The listing builds one solid part. Answer for the finished solid, in the listing's coordinates (mm). Face numbers are marked on the shaded views. A direction names the side the tool comes from. Round coordinates to 2 decimals unless told otherwise and drop trailing zeros. Loops run counter-clockwise (first coordinate to the right, second up) from the corner with the lowest first, then second, coordinate; pieces in that order, holes last. Notation, with made-up numbers: M 29,-13 L 59,-13 A19 ccw 59,3 Z; hole C -23.5,-9.5 d4. An arc over 180 degrees is marked long. Answer as a JSON object with one key per item and string values.
```python
from build123d import *

# Parameters (mm, degrees)
BOX002_W          = 3.6
BOX002_H          = 65
BOX002_DEPTH      = 10
CYLINDER004_R     = 1.8
CYLINDER004_DEPTH = 10
ARRAY_Y_COUNT     = 2
ARRAY_Y_PITCH     = 65
BOX004_W          = 15
BOX004_H          = 29
BOX004_DEPTH      = 10
BOX003_W          = 9.6
BOX003_H          = 65
BOX003_DEPTH      = 4
BOX005_W          = 20
BOX005_H          = 46
BOX005_DEPTH      = 4
CYLINDER006_W     = 23
CYLINDER006_H     = 4
CYLINDER006_ANGLE = 180
CYLINDER005_R     = 4.8
CYLINDER005_DEPTH = 4
ARRAY001_Y_COUNT  = 2
ARRAY001_Y_PITCH  = 65


with BuildPart() as cube002:
    # Box002 → Box002 (new body)
    with BuildSketch(Plane(origin=(-1.8, -32.5, 0), x_dir=(1, 0, 0), z_dir=(0, 0, 1))):
        with Locations((1.8, 32.5)):
            Rectangle(BOX002_W, BOX002_H)
    extrude(amount=BOX002_DEPTH)


with BuildPart() as bolt_hole_fusion:
    # Cylinder004 → Cylinder004 (new body)
    with BuildSketch(Plane.XY):
        Circle(CYLINDER004_R)
    extrude(amount=CYLINDER004_DEPTH)

    # Array Y: bolt hole fusion ×2


with BuildPart() as bolt_hole_fusion_1:
    add(bolt_hole_fusion.part)
    with Locations(*[(0, i * ARRAY_Y_PITCH, 0) for i in range(1, ARRAY_Y_COUNT)]):
        add(bolt_hole_fusion.part)


with BuildPart() as bolt_hole_fusion_2:
    # Array placement: moved
    add(bolt_hole_fusion_1.part.moved(Location((0, -32.5, 0))))

    # Fusion003: union Cube002
    add(cube002.part)


with BuildPart() as extract_fusion:
    # Box004 → Box004 (new body)
    with BuildSketch(Plane(origin=(-8, -14, 0), x_dir=(1, 0, 0), z_dir=(0, 0, 1))):
        with Locations((7.5, 14.5)):
            Rectangle(BOX004_W, BOX004_H)
    extrude(amount=BOX004_DEPTH)

    # Fusion005: union bolt hole fusion
    add(bolt_hole_fusion_2.part)


with BuildPart() as wall_cube:
    # Box003 → Box003 (new body)
    with BuildSketch(Plane(origin=(-4.8, -32.5, 0), x_dir=(1, 0, 0), z_dir=(0, 0, 1))):
        with Locations((4.8, 32.5)):
            Rectangle(BOX003_W, BOX003_H)
    extrude(amount=BOX003_DEPTH)


with BuildPart() as obj1:
    # Box005 → Box005 (new body)
    with BuildSketch(Plane(origin=(-10, -23, 0), x_dir=(1, 0, 0), z_dir=(0, 0, 1))):
        with Locations((10, 23)):
            Rectangle(BOX005_W, BOX005_H)
    extrude(amount=BOX005_DEPTH)


with BuildPart() as cover_cylinder:
    # Cylinder006 → Cylinder006 (revolve)
    with BuildSketch(Plane(origin=(10, 0, 0), x_dir=(0, -1, 0), z_dir=(-1, 0, 0))):
        with Locations((11.5, 2)):
            Rectangle(CYLINDER006_W, CYLINDER006_H)
    revolve(axis=Axis((10, 0, 0), (0, 0, 1)), revolution_arc=CYLINDER006_ANGLE)


with BuildPart() as part_mirroring:
    # Part__Mirroring: instance of cover cylinder
    add(cover_cylinder.part.mirror(Plane(origin=(0, 0, 0), x_dir=(0, -1, 0), z_dir=(1, 0, 0))))


with BuildPart() as microscope_attachment_cut:
    # Cylinder005 → Cylinder005 (new body)
    with BuildSketch(Plane.XY):
        Circle(CYLINDER005_R)
    extrude(amount=CYLINDER005_DEPTH)

    # Array001 Y: microscope attachment cut ×2


with BuildPart() as microscope_attachment_cut_1:
    add(microscope_attachment_cut.part)
    with Locations(*[(0, i * ARRAY001_Y_PITCH, 0) for i in range(1, ARRAY001_Y_COUNT)]):
        add(microscope_attachment_cut.part)


with BuildPart() as microscope_attachment_cut_2:
    # Array001 placement: moved
    add(microscope_attachment_cut_1.part.moved(Location((0, -32.5, 0))))

    # Fusion004: union wall cube, obj1, Part__Mirroring, cover cylinder
    add(wall_cube.part)
    add(obj1.part)
    add(part_mirroring.part)
    add(cover_cylinder.part)

    # Cut001: cut extract fusion
    add(extract_fusion.part, mode=Mode.SUBTRACT)


solid = microscope_attachment_cut_2.part
```
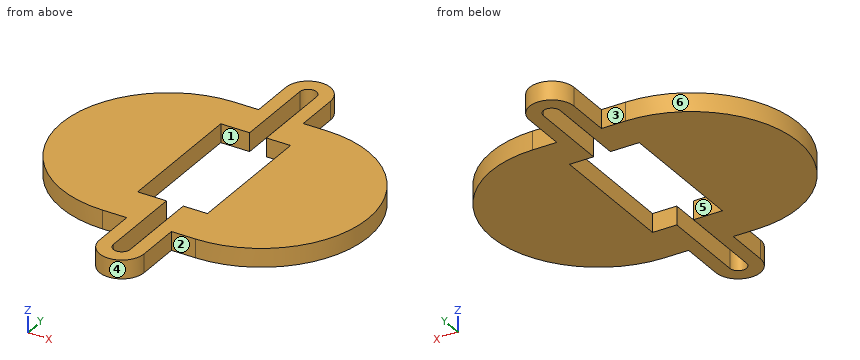
Item 1: Which of the six approach directions +Z, -Z, +X, -X, +Y, -Y give full straight-line access (tool end or side, diameter ignored) to the marked faces 1, 2 and 3?
Values follow:
{"face 1": "+Z, -Z", "face 2": "+Z, -Z, +X, -Y", "face 3": "+Z, -Z, -X, +Y"}
Item 2: The part is cut by section C-C (z = 1.9). Give the vertices of the cut face in (x, y).
Values follow:
{"outline": "M -10,-23 L -4.8,-23 L -4.8,-32.5 A4.8 ccw 4.8,-32.5 L 4.8,-23 L 10,-23 A23 ccw 10,23 L 4.8,23 L 4.8,32.5 A4.8 ccw -4.8,32.5 L -4.8,23 L -10,23 A23 ccw Z; hole M -8,-14 L -1.8,-14 L -1.8,-32.5 A1.8 ccw 1.8,-32.5 L 1.8,-14 L 7,-14 L 7,15 L 1.8,15 L 1.8,32.5 A1.8 ccw -1.8,32.5 L -1.8,15 L -8,15 Z"}
Item 3: The part is cut by section D-D (x = 24.5). Give the vertices of the cut face in (y, z).
Values follow:
{"outline": "M -17.85,0 L 17.85,0 L 17.85,4 L -17.85,4 Z"}
Item 4: Straight lines are drawn through the part: line 1 (X direction, y = 32, z = 1.5); line 2 (Y direction, x = 5, z = 1); line 3 (X direction, y = -15, z = 2.2). For each, find the intervals that lie inside material, in ascending order.
Values follow:
{"line 1": "-4.8 to -1.8, 1.8 to 4.8", "line 2": "-23 to -14, 15 to 23", "line 3": "-27.44 to -1.8, 1.8 to 27.44"}
Item 5: The part is cut by section A-A (y = -31.5). Give the vertices of the cut face in (x, z).
Values follow:
{"outline": "M -4.8,0 L -1.8,0 L -1.8,4 L -4.8,4 Z; M 1.8,0 L 4.8,0 L 4.8,4 L 1.8,4 Z"}
Item 6: Flat-ended cylindrical pins translate along their axes: P1, Ø2, axis at y = -28, z = 1.5, coming from the -X side; P2, Ø2, axis at y = 20, z = 1.5, coming from the -X side; P3, Ø1.2, axis at x = -5, z = 2, coming from the +Y side. Find the tip coordinate at first contact, or state that the pin passes through.
Values follow:
{"P1": "x = -4.8", "P2": "x = -22.96", "P3": "y = 34.42"}
Item 7: Determine the mould class of the marked faces 4, 5 and 6 for opening direction X: released by +X, released by -X, zero draft, split by the parting line, or undercut.
Values follow:
{"face 4": "split by the parting line", "face 5": "undercut", "face 6": "released by -X"}
Item 8: The part is cut by section B-B (x = 0). Give the vertices of the cut face in (y, z).
Values follow:
{"outline": "M -37.3,0 L -34.3,0 L -34.3,4 L -37.3,4 Z; M 34.3,0 L 37.3,0 L 37.3,4 L 34.3,4 Z"}
